from build123d import *

# Parameters (mm, degrees)
SKETCH1_W           = 114.3
SKETCH1_H           = 38.1
BOSS_EXTRUDE1_DEPTH = 25.4
CUT_EXTRUDE1_REACH  = 125.131
SKETCH2_W           = 33.528
SKETCH2_H           = 20.828
CUT_EXTRUDE2_REACH  = 125.131
SKETCH3_R           = 1.778
CUT_EXTRUDE3_REACH  = 125.131
SKETCH4_R           = 1.778
CUT_EXTRUDE4_REACH  = 125.131
SKETCH5_R           = 1.778
SKETCH5_R_2         = 6.35
CUT_EXTRUDE5_REACH  = 125.131
SKETCH6_R           = 1.778
SKETCH6_R_2         = 6.35
CUT_EXTRUDE6_REACH  = 125.131
SKETCH7_R           = 1.778
SKETCH7_R_2         = 6.35
CUT_EXTRUDE7_REACH  = 125.131
SKETCH8_R           = 1.778
SKETCH8_R_2         = 6.35
CUT_EXTRUDE8_REACH  = 125.131
SKETCH9_R           = 1.778
CUT_EXTRUDE9_REACH  = 125.131
SKETCH10_R          = 1.778


with BuildPart() as part:
    # Sketch1 → Boss-Extrude1 (new body)
    with BuildSketch(Plane(origin=(0, 0, 0), x_dir=(1, 0, 0), z_dir=(0, 1, 0))):
        with Locations((-57.15, -19.05)):
            Rectangle(SKETCH1_W, SKETCH1_H)
    extrude(amount=BOSS_EXTRUDE1_DEPTH)

    # Sketch2 → Cut-Extrude1 (cut, up to next)
    with BuildSketch(Plane(origin=(0, 0, 0), x_dir=(0, 0, -1), z_dir=(1, 0, 0)), mode=Mode.PRIVATE) as cut_extrude1_sk1:
        with Locations((-19.05, 12.7)):
            Rectangle(SKETCH2_W, SKETCH2_H)
    cut_extrude1_tool1 = extrude(cut_extrude1_sk1.sketch, amount=-CUT_EXTRUDE1_REACH, mode=Mode.PRIVATE) & part.part
    add(cut_extrude1_tool1.solids().sort_by_distance((0, 12.7, 19.05))[0], mode=Mode.SUBTRACT)

    # Sketch3 → Cut-Extrude2 (cut, up to next)
    with BuildSketch(Plane.XY.offset(38.1), mode=Mode.PRIVATE) as cut_extrude2_sk1:
        with Locations((-2.54, 12.7)):
            Circle(SKETCH3_R)
    cut_extrude2_tool1 = extrude(cut_extrude2_sk1.sketch, amount=-CUT_EXTRUDE2_REACH, mode=Mode.PRIVATE) & part.part
    add(cut_extrude2_tool1.solids().sort_by_distance((-2.54, 12.7, 38.1))[0], mode=Mode.SUBTRACT)

    # Sketch4 → Cut-Extrude3 (cut, up to next)
    with BuildSketch(Plane(origin=(0, 0, 0), x_dir=(-1, 0, 0), z_dir=(0, 0, -1)), mode=Mode.PRIVATE) as cut_extrude3_sk1:
        with Locations(Location((2.54, 12.7, 0), (0, 0, 180))):
            Circle(SKETCH4_R)
    cut_extrude3_tool1 = extrude(cut_extrude3_sk1.sketch, amount=-CUT_EXTRUDE3_REACH, mode=Mode.PRIVATE) & part.part
    add(cut_extrude3_tool1.solids().sort_by_distance((-2.54, 12.7, 0))[0], mode=Mode.SUBTRACT)

    # Sketch5 → Cut-Extrude4 (cut, up to next)
    with BuildSketch(Plane.XY.offset(38.1), mode=Mode.PRIVATE) as cut_extrude4_sk1:
        with Locations((-111.76, 12.7)):
            Circle(SKETCH5_R)
    cut_extrude4_tool1 = extrude(cut_extrude4_sk1.sketch, amount=-CUT_EXTRUDE4_REACH, mode=Mode.PRIVATE) & part.part
    # Sketch5 → Cut-Extrude4 (cut, up to next)
    with BuildSketch(Plane.XY.offset(38.1), mode=Mode.PRIVATE) as cut_extrude4_sk2:
        with Locations((-88.9, 12.7)):
            Circle(SKETCH5_R_2)
    cut_extrude4_tool2 = extrude(cut_extrude4_sk2.sketch, amount=-CUT_EXTRUDE4_REACH, mode=Mode.PRIVATE) & part.part
    # Sketch5 → Cut-Extrude4 (cut, up to next)
    with BuildSketch(Plane.XY.offset(38.1), mode=Mode.PRIVATE) as cut_extrude4_sk3:
        with Locations((-95.814797213, 19.614797213)):
            Circle(SKETCH5_R)
    cut_extrude4_tool3 = extrude(cut_extrude4_sk3.sketch, amount=-CUT_EXTRUDE4_REACH, mode=Mode.PRIVATE) & part.part
    # Sketch5 → Cut-Extrude4 (cut, up to next)
    with BuildSketch(Plane.XY.offset(38.1), mode=Mode.PRIVATE) as cut_extrude4_sk4:
        with Locations((-81.985202787, 19.614797213)):
            Circle(SKETCH5_R)
    cut_extrude4_tool4 = extrude(cut_extrude4_sk4.sketch, amount=-CUT_EXTRUDE4_REACH, mode=Mode.PRIVATE) & part.part
    # Sketch5 → Cut-Extrude4 (cut, up to next)
    with BuildSketch(Plane.XY.offset(38.1), mode=Mode.PRIVATE) as cut_extrude4_sk5:
        with Locations((-95.814797213, 5.785202787)):
            Circle(SKETCH5_R)
    cut_extrude4_tool5 = extrude(cut_extrude4_sk5.sketch, amount=-CUT_EXTRUDE4_REACH, mode=Mode.PRIVATE) & part.part
    # Sketch5 → Cut-Extrude4 (cut, up to next)
    with BuildSketch(Plane.XY.offset(38.1), mode=Mode.PRIVATE) as cut_extrude4_sk6:
        with Locations((-81.985202787, 5.785202787)):
            Circle(SKETCH5_R)
    cut_extrude4_tool6 = extrude(cut_extrude4_sk6.sketch, amount=-CUT_EXTRUDE4_REACH, mode=Mode.PRIVATE) & part.part
    add(cut_extrude4_tool1.solids().sort_by_distance((-111.76, 12.7, 38.1))[0], mode=Mode.SUBTRACT)
    add(cut_extrude4_tool2.solids().sort_by_distance((-88.9, 12.7, 38.1))[0], mode=Mode.SUBTRACT)
    add(cut_extrude4_tool3.solids().sort_by_distance((-95.814797, 19.614797, 38.1))[0], mode=Mode.SUBTRACT)
    add(cut_extrude4_tool4.solids().sort_by_distance((-81.985203, 19.614797, 38.1))[0], mode=Mode.SUBTRACT)
    add(cut_extrude4_tool5.solids().sort_by_distance((-95.814797, 5.785203, 38.1))[0], mode=Mode.SUBTRACT)
    add(cut_extrude4_tool6.solids().sort_by_distance((-81.985203, 5.785203, 38.1))[0], mode=Mode.SUBTRACT)

    # Sketch6 → Cut-Extrude5 (cut, up to next)
    with BuildSketch(Plane(origin=(0, 0, 0), x_dir=(-1, 0, 0), z_dir=(0, 0, -1)), mode=Mode.PRIVATE) as cut_extrude5_sk1:
        with Locations(Location((111.76, 12.7, 0), (0, 0, 180))):
            Circle(SKETCH6_R)
    cut_extrude5_tool1 = extrude(cut_extrude5_sk1.sketch, amount=-CUT_EXTRUDE5_REACH, mode=Mode.PRIVATE) & part.part
    # Sketch6 → Cut-Extrude5 (cut, up to next)
    with BuildSketch(Plane(origin=(0, 0, 0), x_dir=(-1, 0, 0), z_dir=(0, 0, -1)), mode=Mode.PRIVATE) as cut_extrude5_sk2:
        with Locations(Location((88.9, 12.7, 0), (0, 0, 180))):
            Circle(SKETCH6_R_2)
    cut_extrude5_tool2 = extrude(cut_extrude5_sk2.sketch, amount=-CUT_EXTRUDE5_REACH, mode=Mode.PRIVATE) & part.part
    # Sketch6 → Cut-Extrude5 (cut, up to next)
    with BuildSketch(Plane(origin=(0, 0, 0), x_dir=(-1, 0, 0), z_dir=(0, 0, -1)), mode=Mode.PRIVATE) as cut_extrude5_sk3:
        with Locations(Location((81.985202787, 19.614797213, 0), (0, 0, 180))):
            Circle(SKETCH6_R)
    cut_extrude5_tool3 = extrude(cut_extrude5_sk3.sketch, amount=-CUT_EXTRUDE5_REACH, mode=Mode.PRIVATE) & part.part
    # Sketch6 → Cut-Extrude5 (cut, up to next)
    with BuildSketch(Plane(origin=(0, 0, 0), x_dir=(-1, 0, 0), z_dir=(0, 0, -1)), mode=Mode.PRIVATE) as cut_extrude5_sk4:
        with Locations(Location((95.814797213, 19.614797213, 0), (0, 0, 180))):
            Circle(SKETCH6_R)
    cut_extrude5_tool4 = extrude(cut_extrude5_sk4.sketch, amount=-CUT_EXTRUDE5_REACH, mode=Mode.PRIVATE) & part.part
    # Sketch6 → Cut-Extrude5 (cut, up to next)
    with BuildSketch(Plane(origin=(0, 0, 0), x_dir=(-1, 0, 0), z_dir=(0, 0, -1)), mode=Mode.PRIVATE) as cut_extrude5_sk5:
        with Locations(Location((95.814797213, 5.785202787, 0), (0, 0, 180))):
            Circle(SKETCH6_R)
    cut_extrude5_tool5 = extrude(cut_extrude5_sk5.sketch, amount=-CUT_EXTRUDE5_REACH, mode=Mode.PRIVATE) & part.part
    # Sketch6 → Cut-Extrude5 (cut, up to next)
    with BuildSketch(Plane(origin=(0, 0, 0), x_dir=(-1, 0, 0), z_dir=(0, 0, -1)), mode=Mode.PRIVATE) as cut_extrude5_sk6:
        with Locations(Location((81.985202787, 5.785202787, 0), (0, 0, 180))):
            Circle(SKETCH6_R)
    cut_extrude5_tool6 = extrude(cut_extrude5_sk6.sketch, amount=-CUT_EXTRUDE5_REACH, mode=Mode.PRIVATE) & part.part
    add(cut_extrude5_tool1.solids().sort_by_distance((-111.76, 12.7, 0))[0], mode=Mode.SUBTRACT)
    add(cut_extrude5_tool2.solids().sort_by_distance((-88.9, 12.7, 0))[0], mode=Mode.SUBTRACT)
    add(cut_extrude5_tool3.solids().sort_by_distance((-81.985203, 19.614797, 0))[0], mode=Mode.SUBTRACT)
    add(cut_extrude5_tool4.solids().sort_by_distance((-95.814797, 19.614797, 0))[0], mode=Mode.SUBTRACT)
    add(cut_extrude5_tool5.solids().sort_by_distance((-95.814797, 5.785203, 0))[0], mode=Mode.SUBTRACT)
    add(cut_extrude5_tool6.solids().sort_by_distance((-81.985203, 5.785203, 0))[0], mode=Mode.SUBTRACT)

    # Sketch7 → Cut-Extrude6 (cut, up to next)
    with BuildSketch(Plane(origin=(0, 25.4, 0), x_dir=(1, 0, 0), z_dir=(0, 1, 0)), mode=Mode.PRIVATE) as cut_extrude6_sk1:
        with Locations(Location((-111.76, -19.05, 0), (0, 0, 270))):
            Circle(SKETCH7_R)
    cut_extrude6_tool1 = extrude(cut_extrude6_sk1.sketch, amount=-CUT_EXTRUDE6_REACH, mode=Mode.PRIVATE) & part.part
    # Sketch7 → Cut-Extrude6 (cut, up to next)
    with BuildSketch(Plane(origin=(0, 25.4, 0), x_dir=(1, 0, 0), z_dir=(0, 1, 0)), mode=Mode.PRIVATE) as cut_extrude6_sk2:
        with Locations(Location((-88.9, -19.05, 0), (0, 0, 270))):
            Circle(SKETCH7_R_2)
    cut_extrude6_tool2 = extrude(cut_extrude6_sk2.sketch, amount=-CUT_EXTRUDE6_REACH, mode=Mode.PRIVATE) & part.part
    add(cut_extrude6_tool1.solids().sort_by_distance((-111.76, 25.4, 19.05))[0], mode=Mode.SUBTRACT)
    add(cut_extrude6_tool2.solids().sort_by_distance((-88.9, 25.4, 19.05))[0], mode=Mode.SUBTRACT)

    # Sketch8 → Cut-Extrude7 (cut, up to next)
    with BuildSketch(Plane.XZ, mode=Mode.PRIVATE) as cut_extrude7_sk1:
        with Locations(Location((-111.76, 19.05, 0), (0, 0, 90))):
            Circle(SKETCH8_R)
    cut_extrude7_tool1 = extrude(cut_extrude7_sk1.sketch, amount=-CUT_EXTRUDE7_REACH, mode=Mode.PRIVATE) & part.part
    # Sketch8 → Cut-Extrude7 (cut, up to next)
    with BuildSketch(Plane.XZ, mode=Mode.PRIVATE) as cut_extrude7_sk2:
        with Locations(Location((-88.9, 19.05, 0), (0, 0, 90))):
            Circle(SKETCH8_R_2)
    cut_extrude7_tool2 = extrude(cut_extrude7_sk2.sketch, amount=-CUT_EXTRUDE7_REACH, mode=Mode.PRIVATE) & part.part
    add(cut_extrude7_tool1.solids().sort_by_distance((-111.76, 0, 19.05))[0], mode=Mode.SUBTRACT)
    add(cut_extrude7_tool2.solids().sort_by_distance((-88.9, 0, 19.05))[0], mode=Mode.SUBTRACT)

    # Sketch9 → Cut-Extrude8 (cut, up to next)
    with BuildSketch(Plane(origin=(0, 25.4, 0), x_dir=(1, 0, 0), z_dir=(0, 1, 0)), mode=Mode.PRIVATE) as cut_extrude8_sk1:
        with Locations(Location((-2.54, -19.05, 0), (0, 0, 270))):
            Circle(SKETCH9_R)
    cut_extrude8_tool1 = extrude(cut_extrude8_sk1.sketch, amount=-CUT_EXTRUDE8_REACH, mode=Mode.PRIVATE) & part.part
    add(cut_extrude8_tool1.solids().sort_by_distance((-2.54, 25.4, 19.05))[0], mode=Mode.SUBTRACT)

    # Sketch10 → Cut-Extrude9 (cut, up to next)
    with BuildSketch(Plane(origin=(0, 0, 0), x_dir=(-1, 0, 0), z_dir=(0, -1, 0)), mode=Mode.PRIVATE) as cut_extrude9_sk1:
        with Locations(Location((2.54, -19.05, 0), (0, 0, 270))):
            Circle(SKETCH10_R)
    cut_extrude9_tool1 = extrude(cut_extrude9_sk1.sketch, amount=-CUT_EXTRUDE9_REACH, mode=Mode.PRIVATE) & part.part
    add(cut_extrude9_tool1.solids().sort_by_distance((-2.54, 0, 19.05))[0], mode=Mode.SUBTRACT)


solid = part.part
The model under review builds one solid part; all positions refer to its coordinate system, in mm. A direction names the side the tool comes from. Give positions to 0.01 mm unless a question says otherwise; leave off trailing zeros. Write each loop counter-clockwise with the first axis right and the second up, starting at its lowest first coordinate (ties: lowest second). Pieces come first, ordered by that corner, then holes.
1. For P1, Ø4.5, axis at x = -95.81, y = 5.79, coming from the -Z side, flat-tipped, find the tip position at first contact; note if it passes through.
2. Draft analysis for pull direction X (two halves, no side actions). For faces 3 (the cylindrical face through (-97.59, 5.71, 1.13)), 4 (the flat face through (0, 1, 19)), 5 (the flat face through (-56, 2.286, 19)), state which applies: +X half, -X half, draft (parallel to the pull), parting line (faces both ways), or undercut.
3. Add section A-A, the plane x = -2.54. Write out the cut boundary in (y, z), plus the area to 3 significant figures.
4. Tool access review of faces 1 (the flat face through (-114.3, 1, 19)), 2 (the flat face through (-56, 23.114, 19)): name each direction out of +Z, -Z, +X, -X, +Y, -Y from which nothing blocks a thin tool from reaching the whole face with its end or side.
5. Wall thickness on L1, parallel to Y at x = -45.5, z = 24.5; L2, parallel to Z at x = -57.5, y = 10.5; L3, parallel to Z at x = -111.76, y = 23.8: over which ranges is each line inside the solid? List them lowest first.
6. Add section B-B, the plane z = 7. Write out the cut boundary in (x, y).
7. Add section C-C, the plane z = 19.05. Count the separate pieces of the cut face and the enclosed holes in it, plus the area to 3 significant figures.
8. Add section D-D, the plane y = 9.25. Write out the cut boundary in (x, z).
Worked answers:
1. P1: stops at z = 0
2. face 3: undercut
2. face 4: +X half
2. face 5: draft
3. outline: (0, 0) - (10.92, 0) - (10.92, 2.29) - (2.29, 2.29) - (2.29, 17.27) - (0, 17.27) - close; (0, 20.83) - (2.29, 20.83) - (2.29, 35.81) - (10.92, 35.81) - (10.92, 38.1) - (0, 38.1) - close; (14.48, 0) - (25.4, 0) - (25.4, 17.27) - (23.11, 17.27) - (23.11, 2.29) - (14.48, 2.29) - close; (14.48, 35.81) - (23.11, 35.81) - (23.11, 20.83) - (25.4, 20.83) - (25.4, 38.1) - (14.48, 38.1) - close
3. area: 237 mm2
4. face 1: +Z, -Z, -X, +Y, -Y
4. face 2: +X, -X
5. L1: y = 0 to 2.29, 23.11 to 25.4
5. L2: z = 0 to 2.29, 35.81 to 38.1
5. L3: z = 0 to 17.27, 20.83 to 38.1
6. outline: (-114.3, 0) - (0, 0) - (0, 2.29) - (-114.3, 2.29) - close; (-114.3, 23.11) - (0, 23.11) - (0, 25.4) - (-114.3, 25.4) - close
7. separate pieces: 8
7. enclosed holes: 0
7. area: 432 mm2
8. outline: (-114.3, 0) - (-94.23, 0) - (-94.23, 2.29) - (-114.3, 2.29) - close; (-114.3, 35.81) - (-94.23, 35.81) - (-94.23, 38.1) - (-114.3, 38.1) - close; (-83.57, 0) - (0, 0) - (0, 2.29) - (-83.57, 2.29) - close; (-83.57, 35.81) - (0, 35.81) - (0, 38.1) - (-83.57, 38.1) - close
